from build123d import *

# Parameters (mm, degrees)
MODEL_R                 = 1.5
SALIENTE_EXTRUIR1_DEPTH = 3


with BuildPart() as part:
    # Model → Saliente-Extruir1 (new body)
    with BuildSketch(Plane.XY):
        with BuildLine():
            Line((201.097853309, 264.646547335), (180.097853309, 264.646547335))
            Line((180.097853309, 264.646547335), (180.097853309, 282.646547335))
            Line((180.097853309, 282.646547335), (192.097853309, 282.646547335))
            ThreePointArc((192.097853309, 282.646547335), (192.676448554, 282.540050724), (193.179205728, 282.234519695))
            Line((193.179205728, 282.234519695), (204.092367701, 272.505547716))
            ThreePointArc((204.092367701, 272.505547716), (205.302939617, 267.544283579), (201.097853309, 264.646547335))
        make_face()
        with Locations((201.097853309, 269.146547335)):
            Circle(MODEL_R, mode=Mode.SUBTRACT)
        with BuildLine():
            Line((183.722853309, 265.896547335), (185.472853309, 265.896547335))
            ThreePointArc((185.472853309, 265.896547335), (186.003183395, 266.116217249), (186.222853309, 266.646547335))
            Line((186.222853309, 266.646547335), (186.222853309, 271.646547335))
            ThreePointArc((186.222853309, 271.646547335), (186.003183395, 272.176877421), (185.472853309, 272.396547335))
            Line((185.472853309, 272.396547335), (183.722853309, 272.396547335))
            ThreePointArc((183.722853309, 272.396547335), (183.192523223, 272.176877421), (182.972853309, 271.646547335))
            Line((182.972853309, 271.646547335), (182.972853309, 266.646547335))
            ThreePointArc((182.972853309, 266.646547335), (183.192523223, 266.116217249), (183.722853309, 265.896547335))
        make_face(mode=Mode.SUBTRACT)
        with BuildLine():
            Line((183.722853309, 274.895968764), (185.472853309, 274.895968764))
            ThreePointArc((185.472853309, 274.895968764), (186.003183395, 275.115638678), (186.222853309, 275.645968764))
            Line((186.222853309, 275.645968764), (186.222853309, 280.645968764))
            ThreePointArc((186.222853309, 280.645968764), (186.003183395, 281.17629885), (185.472853309, 281.395968764))
            Line((185.472853309, 281.395968764), (183.722853309, 281.395968764))
            ThreePointArc((183.722853309, 281.395968764), (183.192523223, 281.17629885), (182.972853309, 280.645968764))
            Line((182.972853309, 280.645968764), (182.972853309, 275.645968764))
            ThreePointArc((182.972853309, 275.645968764), (183.192523223, 275.115638678), (183.722853309, 274.895968764))
        make_face(mode=Mode.SUBTRACT)
    extrude(amount=SALIENTE_EXTRUIR1_DEPTH)


solid = part.part
Geometry check sheet. Reference: the model listing, model coordinates, mm. A direction names the side the tool comes from. Round coordinates to 2 decimals unless told otherwise and drop trailing zeros. Write each loop counter-clockwise with the first axis right and the second up, starting at its lowest first coordinate (ties: lowest second). Pieces come first, ordered by that corner, then holes. Notation, with made-up numbers: (56.5, 67) - (113.5, 67) arc R21 ccw to (113.5, 99) - close; hole circle Ø3 at (82.25, 51.25). An arc over 180 degrees is marked (long way). One line per item, written item: value.
1. Set-up check for faces 1 (the face through (198.6, 277.4, 1.5)), 2 (the face through (186.223, 278, 1)): record each of +Z, -Z, +X, -X, +Y, -Y from which the full face is reachable in a straight line by a thin tool's end or side.
The answers:
face 1: +Z, -Z, +X, +Y
face 2: +Z, -Z
2. Scan lines: L1, parallel to X at y = 270.25, z = 1.3; L2, parallel to X at y = 272, z = 2.8; L3, parallel to X at y = 270, z = 2.5. Record each from-to range of solid material in increasing order.
The answers:
L1: x = 180.1 to 182.97, 186.22 to 200.08, 202.11 to 205.46
L2: x = 180.1 to 183.06, 186.13 to 204.58
L3: x = 180.1 to 182.97, 186.22 to 199.86, 202.33 to 205.52
3. Cross-section at A-A on y = 269.75. Record the boundary of the cut face in (x, z).
The answers:
outline: (180.1, 0) - (182.97, 0) - (182.97, 3) - (180.1, 3) - close; (186.22, 0) - (199.72, 0) - (199.72, 3) - (186.22, 3) - close; (202.47, 0) - (205.56, 0) - (205.56, 3) - (202.47, 3) - close
4. Cross-section at C-C on y = 267. Record the boundary of the cut face in (x, z).
The answers:
outline: (180.1, 0) - (182.97, 0) - (182.97, 3) - (180.1, 3) - close; (186.22, 0) - (205.05, 0) - (205.05, 3) - (186.22, 3) - close
5. Mould release check, pull along Y, two halves, no side actions. Record for faces 3 (the face through (185, 265.897, 1)), 4 (the face through (190, 274, 0)), 5 (the face through (192.669, 282.543, 1.479)): released by +Y, released by -Y, zero draft, split by the parting line, or undercut.
The answers:
face 3: undercut
face 4: zero draft
face 5: released by +Y
6. Cross-section at B-B on z = 1.25. Record the boundary of the cut face in (x, y) (3 decimals).
The answers:
outline: (180.098, 264.647) - (201.098, 264.647) arc R4.5 ccw to (204.092, 272.506) - (193.179, 282.235) arc R1.625 ccw to (192.098, 282.647) - (180.098, 282.647) - close; hole (182.973, 266.647) arc R0.75 ccw to (183.723, 265.897) - (185.473, 265.897) arc R0.75 ccw to (186.223, 266.647) - (186.223, 271.647) arc R0.75 ccw to (185.473, 272.397) - (183.723, 272.397) arc R0.75 ccw to (182.973, 271.647) - close; hole (182.973, 275.646) arc R0.75 ccw to (183.723, 274.896) - (185.473, 274.896) arc R0.75 ccw to (186.223, 275.646) - (186.223, 280.646) arc R0.75 ccw to (185.473, 281.396) - (183.723, 281.396) arc R0.75 ccw to (182.973, 280.646) - close; hole circle Ø3 at (201.098, 269.147)
7. Cross-section at D-D on x = 198. Record the boundary of the cut face in (y, z), and give its area (3 significant figures).
The answers:
outline: (264.65, 0) - (277.94, 0) - (277.94, 3) - (264.65, 3) - close
area: 39.9 mm^2
